from build123d import *

# Parameters (mm, degrees)
BOSS_EXTRU_1_DEPTH           = 0.1
BOSS_EXTRU_1_DEPTH_BACK      = 6.9
ESQUISSE1_R                  = 25
ESQUISSE1_R_2                = 1.7
ESQUISSE2_W                  = 37
ESQUISSE2_H                  = 8
ENL_V_MAT_EXTRU_1_DEPTH      = 37.041642582
ENL_V_MAT_EXTRU_3_DEPTH      = 51.801015595
ENL_V_MAT_EXTRU_3_DEPTH_BACK = 51.801015595
ESQUISSE3_W                  = 2.84
ESQUISSE3_H                  = 14


with BuildPart() as part:
    # Esquisse1 → Boss.-Extru.1 (new, two sides: drawn at the far end of the back side and taken through both)
    with BuildSketch(Plane.XY.offset(-BOSS_EXTRU_1_DEPTH_BACK)):
        Circle(ESQUISSE1_R)
        with Locations((-13.435028843, 13.435028843)):
            Circle(ESQUISSE1_R_2, mode=Mode.SUBTRACT)
        with Locations((13.435028843, 13.435028843)):
            Circle(ESQUISSE1_R_2, mode=Mode.SUBTRACT)
        with Locations((13.435028843, -13.435028843)):
            Circle(ESQUISSE1_R_2, mode=Mode.SUBTRACT)
        with Locations((-13.435028843, -13.435028843)):
            Circle(ESQUISSE1_R_2, mode=Mode.SUBTRACT)
    extrude(amount=BOSS_EXTRU_1_DEPTH + BOSS_EXTRU_1_DEPTH_BACK)

    # Esquisse2 → Enlèv. mat.-Extru.1 (cut, through all)
    with BuildSketch(Plane.XY.offset(0.1)):
        Rectangle(ESQUISSE2_W, ESQUISSE2_H)
    extrude(amount=-ENL_V_MAT_EXTRU_1_DEPTH, mode=Mode.SUBTRACT)

    # Esquisse3 → Enlèv. mat.-Extru.3 (cut, two sides: drawn at the far end of the back side and taken through both)
    with BuildSketch(Plane(origin=(18.5, 0, 1.068261133), x_dir=(0, 0, 1), z_dir=(-1, 0, 0)).offset(-ENL_V_MAT_EXTRU_3_DEPTH_BACK)):
        with Locations((-1.545739837, -0.037482161)):
            Rectangle(ESQUISSE3_W, ESQUISSE3_H)
    extrude(amount=ENL_V_MAT_EXTRU_3_DEPTH + ENL_V_MAT_EXTRU_3_DEPTH_BACK, mode=Mode.SUBTRACT)


solid = part.part
Build history of the part. All positions in model axes, mm. A direction names the side the tool comes from. Coordinates: 2 decimals unless noted, no trailing zeros. Order: outer loops, then holes, each group sorted by start corner. A loop starts at its lowest first (then second) coordinate and runs counter-clockwise, first axis right, second up. Notation, with made-up numbers: M 56.5,7.25 L 77.5,7.25 A27 cw 77.5,38.25 Z; hole C 16.5,71 d9. An arc over 180 degrees is marked long. One line per question, with ' | ' between items. Start each with the question number.
Q1. 3-axis set-ups, long thin cutter, end or side, ignore diameter. For faces 5 (the face through (0, -4, -4)), 6 (the face through (0, 6.963, -1)), 7 (the face through (0, -14, 0.1)): which of +Z, -Z, +X, -X, +Y, -Y reach the whole face in a straight line?
Q2. Saw through at C-C (x = -13). List the corners of the cut face in (y, z), then the cut area to 3 significant figures.
Q3. Two-plate mould, pull along X, no slides. Class faces 1 (the face through (23.846, 7.509, -3.449)), 2 (the face through (18.5, 0, -4)), 3 (the face through (14.219, -14.943, -3.449)), 4 (the face through (0, -7.037, -1)): +X half, -X half, draft (parallel to the pull), parting line (faces both ways), or undercut.
Q4. Flat gauge pins, fed straight in: pin 1 Ø1.5 at (y, z) = (-2, -5) entering from +X; pin 2 Ø4 at (x, z) = (-4, -4.5) entering from -Y; pin 3 Ø0.6 at (x, z) = (-4.5, -0.5) entering from -Y. Where does each tip first touch, or does it go through?
Q5. Saw through at A-A (x = 0). List the corners of the cut face in (y, z).
Q6. Saw through at B-B (y = 0). List the corners of the cut face in (x, z).
Q7. Saw through at D-D (z = -5.5). List the corners of the cut face in (x, y), then the cut area to 3 significant figures.
Q8. Probe L1, parallel to X at y = 13, z = -1.25; L2, parallel to X at y = 7, z = -5.75; L3, parallel to Y at x = -8.5, z = -3.5. List the from-to ranges inside material, lowest first. Write a range as from..to.
Check values:
1) face 5: +Z, -Z | face 6: +Z, +X, -X | face 7: +Z, +X, -X, +Y, -Y
2) outline: M -21.35,-6.9 L -15.08,-6.9 L -15.08,0.1 L -21.35,0.1 Z; M -11.79,-6.9 L -4,-6.9 L -4,-1.9 L -7.04,-1.9 L -7.04,0.1 L -11.79,0.1 Z; M 4,-6.9 L 11.79,-6.9 L 11.79,0.1 L 6.96,0.1 L 6.96,-1.9 L 4,-1.9 Z; M 15.08,-6.9 L 21.35,-6.9 L 21.35,0.1 L 15.08,0.1 Z | area: 185 mm2
3) face 1: parting line | face 2: undercut | face 3: undercut | face 4: draft
4) pin 1: stops at x = 24.97 | pin 2: stops at y = -24.92 | pin 3: stops at y = -24.64
5) outline: M -25,-6.9 L -4,-6.9 L -4,-1.9 L -7.04,-1.9 L -7.04,0.1 L -25,0.1 Z; M 4,-6.9 L 25,-6.9 L 25,0.1 L 6.96,0.1 L 6.96,-1.9 L 4,-1.9 Z
6) outline: M -25,-6.9 L -18.5,-6.9 L -18.5,-1.9 L -25,-1.9 Z; M 18.5,-6.9 L 25,-6.9 L 25,-1.9 L 18.5,-1.9 Z
7) outline: C 0,0 d50; hole M -18.5,-4 L 18.5,-4 L 18.5,4 L -18.5,4 Z; hole C -13.44,-13.44 d3.4; hole C -13.44,13.44 d3.4; hole C 13.44,-13.44 d3.4; hole C 13.44,13.44 d3.4 | area: 1,630 mm2
8) L1: x = -21.35..-15.08, -11.79..11.79, 15.08..21.35 | L2: x = -24..24 | L3: y = -23.51..-4, 4..23.51
